Design review of the part shown in the three views and the two pictorial views. Dimensions are in mm from the part's minimum x, y and z. Give positions to 0.01 mm unless a question says otherwise; leave off trailing zeros. Loops run counter-clockwise (first coordinate to the right, second up) from the corner with the lowest first, then second, coordinate; pieces in that order, holes last.
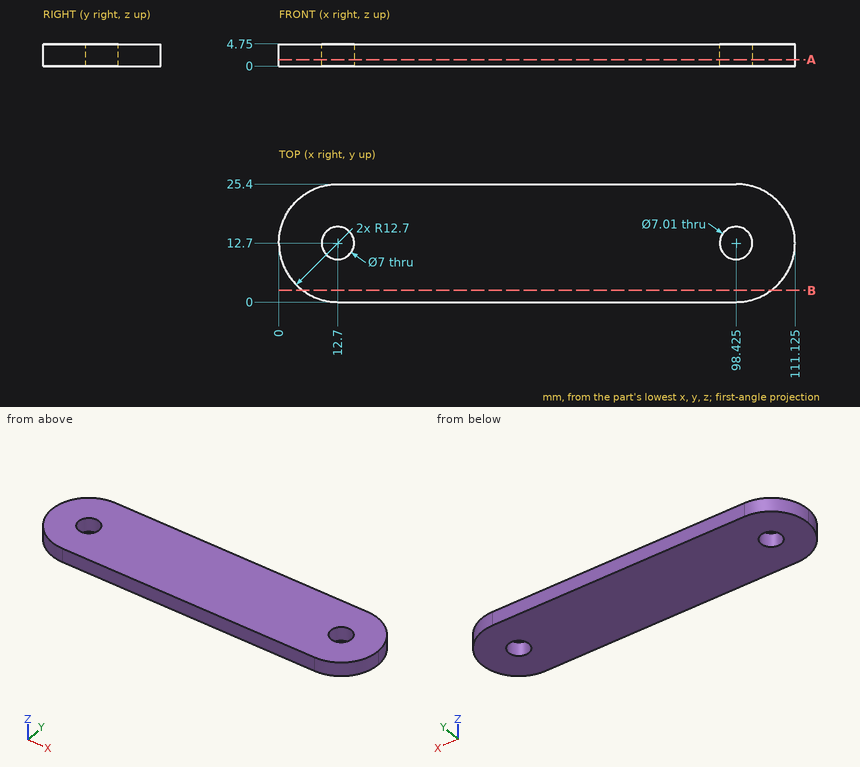
Q1. Take a section at A-A (z = 1.4). Give the number of separate pieces and of enclosed holes in the cut face, plus the area to 3 significant figures.
Results:
separate pieces: 1
enclosed holes: 2
area: 2,610 mm2
Q2. Take a section at B-B (y = 2.5). Give the boundary of the cut face in (x, z).
Results:
outline: (5.13, 0) - (105.99, 0) - (105.99, 4.75) - (5.13, 4.75) - close
Q3. Wall thickness on line 1 (Y direction, x = 12.7, z = 1.7); line 2 (X direction, y = 2, z = 3.9) (1 decimal); line 3 (X direction, y = 21.75, z = 4.05) (1 decimal): over which ranges is each line inside the solid? List them lowest first.
Results:
line 1: y = 0 to 9.2, 16.2 to 25.4
line 2: x = 5.9 to 105.3
line 3: x = 3.8 to 107.3
